Geometry: final body of the model. Coordinates: model frame, mm. Give positions to 0.01 mm unless a question says otherwise; leave off trailing zeros.
Q1. Pin query (flat end, axial travel): pin 1 Ø9.5 at (x, z) = (-23.5, 2) entering from +Y; pin 2 Ø4 at (x, z) = (-119, -72) entering from +Y; pin 3 Ø8 at (x, z) = (-52.5, -52) entering from +Y. Return the tip coordinate at first contact, or that it passes through.
Q2. Line query: line 1 (Y direction, x = -32, z = 112.5); line 2 (Z direction, x = -33, y = 17); line 3 (X direction, y = 15.25, z = -9). Output: solid intervals per line, ascending.
Q3. Mould query, pull axis Z, two halves, no side actions, for faces 1 (the flat face through (-24, 6.483, 3)), 2 (the cylindrical face through (-146.173, 13.385, 17.656)), 3 (the conical face through (-25.989, 10.656, -10.532)). Classes: +Z half, -Z half, draft (parallel to the pull), parting line (faces both ways), or undercut.
from build123d import *


with BuildPart() as part:
    # Sketch1 → Revolve1 (revolve)
    with BuildSketch(Plane(origin=(0, 0, 1.383780883), x_dir=(0, -1, 0), z_dir=(0, 0, 1)), mode=Mode.PRIVATE) as revolve1_sk:
        with BuildLine():
            Line((-6.482641531, -22.236737445), (-16.482641531, -22.236737445))
            Line((-16.482641531, -22.236737445), (-16.482641531, -16.236737445))
            ThreePointArc((-16.482641531, -16.236737445), (-12.404820423, -15.119424058), (-9.466050343, -12.079581198))
            Line((-9.466050343, -12.079581198), (-28.482641531, 25.263262555))
            ThreePointArc((-28.482641531, 25.263262555), (-28.968073531, 28.408526495), (-28.482641531, 31.553790435))
            ThreePointArc((-28.482641531, 31.553790435), (-22.494411783, 57.164168196), (-20.482641531, 83.388262555))
            Line((-20.482641531, 83.388262555), (-20.482641531, 102.763262555))
            Line((-20.482641531, 102.763262555), (-6.482641531, 102.763262555))
            Line((-6.482641531, 102.763262555), (-6.482641531, -22.236737445))
        make_face()
    revolve(revolve1_sk.sketch.rotate(Axis((-22.236737445, 6.482641531, 1.383780883), (0, 1, 0)), 90), axis=Axis((-22.236737445, 6.482641531, 1.383780883), (0, 1, 0)))


solid = part.part
Computed:
1. pin 1: stops at y = 16.48
1. pin 2: stops at y = 20.48
1. pin 3: stops at y = 27.39
2. line 1: y = 6.48 to 20.48
2. line 2: z = -123.15 to -21.13, 23.89 to 125.92
2. line 3: x = -146.8 to -41.08, -3.39 to 102.33
3. face 1: draft
3. face 2: parting line
3. face 3: undercut
